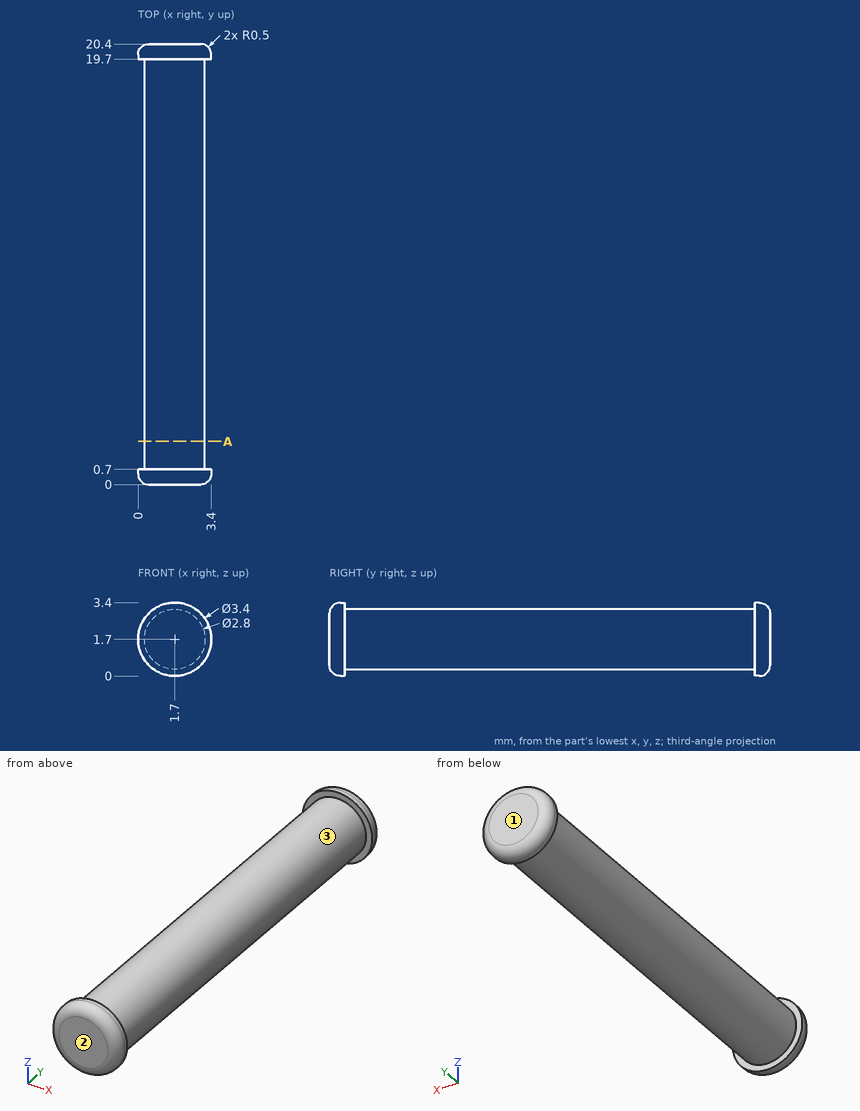
The drawing under review shows one solid part. Ordinate dimensions are in mm from its lowest x, y, z. Round coordinates to 2 decimals unless told otherwise and drop trailing zeros. Write each loop counter-clockwise with the first axis right and the second up, starting at its lowest first coordinate (ties: lowest second). Pieces come first, ordered by that corner, then holes. Notation, with made-up numbers: (23, 44) - (70, 44) arc R27 ccw to (70, 65) - close; hole circle Ø7 at (54, 5.5). An arc over 180 degrees is marked (long way). Use one line per item in the form item = value.
Q1. For line 1 (Y direction, x = 3.25, z = 1.95); line 2 (Y direction, x = 2, z = 0.25); line 3 (Z direction, x = 1.55, y = 3.75), list the stretches that pass through material, from the lowest coordinate up. Write a range as [from, to].
Answer key:
line_1 = [0.16, 0.7], [19.7, 20.24]
line_2 = [0.09, 0.7], [19.7, 20.31]
line_3 = [0.31, 3.09]
Q2. Insertion check: pin 1 Ø1.5 at (x, y) = (1.5, 7) entering from +Z. The pin has a flat end and moves straight along its axis. Give the tip position at first contact, or say it passes through.
Answer key:
pin_1 = 3.1
Q3. Draft analysis for pull direction Y (two halves, no side actions). For the marked faces 1, 2 and 3, state which applies: +Y half, -Y half, draft (parallel to the pull), parting line (faces both ways), or undercut.
Answer key:
face_1 = +Y half
face_2 = -Y half
face_3 = undercut
Q4. Consider section A-A (y = 2). State the section outline as (x, z) points.
Answer key:
outline = circle Ø2.8 at (1.7, 1.7)
